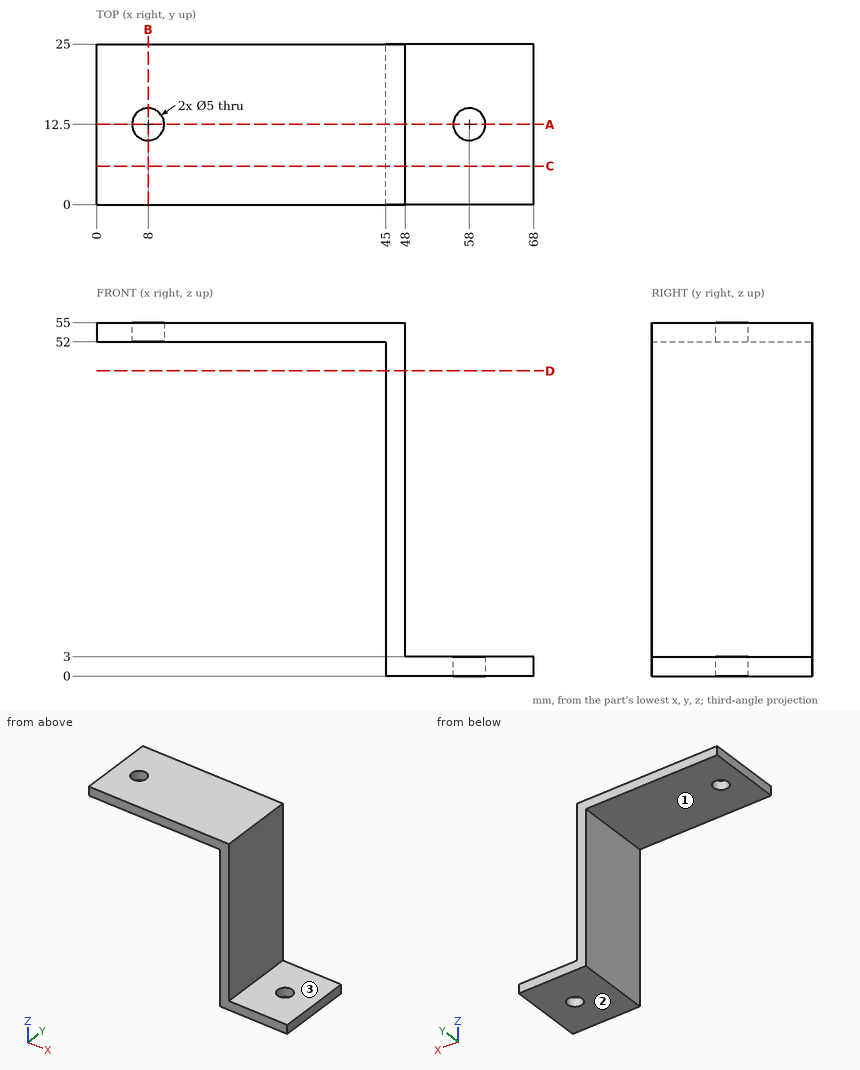
The drawing under review shows one solid part. Ordinate dimensions are in mm from its lowest x, y, z. A direction names the side the tool comes from. Round coordinates to 2 decimals unless told otherwise and drop trailing zeros. Loops run counter-clockwise (first coordinate to the right, second up) from the corner with the lowest first, then second, coordinate; pieces in that order, holes last. Notation, with made-up numbers: (35, 2.25) - (47, 2.25) arc R16 cw to (47, 23.25) - close; hole circle Ø5 at (-23, 38.25). An arc over 180 degrees is marked (long way). Put each result on its own line as item: value. Start each with the question number.
1. Consider section C-C on y = 6. State the section outline as (x, z) points.
2. Consider section D-D on z = 47.5. State the section outline as (x, y) points.
3. For probe 1 along Y at (x, z) = (8, 54.3); probe 2 along X at (y, z) = (13.75, 37); probe 3 along Z at (x, y) = (12, 2.5), list the stretches that pass through material, from the lowest coordinate up. Write a range as [from, to].
4. Consider section B-B on x = 8. State the section outline as (y, z) points, plus the area to 3 significant figures.
5. For the marked faces 1, 2 and 3, list the 3-axis set-ups (+Z, -Z, +X, -X, +Y, -Y) from which the entire face can be reached by the end or side of a thin tool; tool diameter is ignored.
6. Insertion check: P1, Ø12.5, axis at x = 16.5, y = 15, coming from the -Z side; P2, Ø4, axis at y = 5.5, z = 11.5, coming from the +X side; P3, Ø4.5, axis at x = 58, y = 12.5, coming from the -Z side; P4, Ø4, axis at x = 43.5, y = 6, coming from the -Z side. Each pin has a flat end and moves straight along its axis. Give the tip position at first contact, or say it passes through.
7. Consider section A-A on y = 12.5. State the section outline as (x, z) points, plus the area to 3 significant figures.
Result sheet:
1. outline: (0, 52) - (45, 52) - (45, 0) - (68, 0) - (68, 3) - (48, 3) - (48, 55) - (0, 55) - close
2. outline: (45, 0) - (48, 0) - (48, 25) - (45, 25) - close
3. probe 1: [0, 10], [15, 25]
3. probe 2: [45, 48]
3. probe 3: [52, 55]
4. outline: (0, 52) - (10, 52) - (10, 55) - (0, 55) - close; (15, 52) - (25, 52) - (25, 55) - (15, 55) - close
4. area: 60.0 mm^2
5. face 1: -Z, -X, +Y, -Y
5. face 2: -Z, +X, -X, +Y, -Y
5. face 3: +Z, +X, +Y, -Y
6. P1: z = 52
6. P2: x = 48
6. P3: through
6. P4: z = 0
7. outline: (0, 52) - (5.5, 52) - (5.5, 55) - (0, 55) - close; (10.5, 52) - (45, 52) - (45, 0) - (55.5, 0) - (55.5, 3) - (48, 3) - (48, 55) - (10.5, 55) - close; (60.5, 0) - (68, 0) - (68, 3) - (60.5, 3) - close
7. area: 330 mm^2
